Source: CAD feature listing. Evaluate the final solid. Frame: model axes, mm. A direction names the side the tool comes from. Round coordinates to 2 decimals unless told otherwise and drop trailing zeros. Loops run counter-clockwise (first coordinate to the right, second up) from the corner with the lowest first, then second, coordinate; pieces in that order, holes last.
(1) Section A-A, the plane y = 5. Return the cut outline in (x, z).
(2) First-contact query: pin 1 Ø6 at (x, z) = (18.5, 3) entering from +Y; pin 2 Ø4 at (x, y) = (53, 18) entering from +Z. Flat tips, straight axial feed; report the tip coordinate or a pass-through.
(3) Section C-C, the plane y = 36. Return the cut outline in (x, z), plus the area to 3 significant figures.
(4) Section B-B, the plane x = 54. Return the cut outline in (y, z).
(5) Material intervals for probe 1 along X at (y, z) = (50.25, 6); probe 2 along X at (y, z) = (19.5, 10.25); probe 3 along X at (y, z) = (51, 6), sorted ascending.
(6) Mould query, pull axis Z, two halves, no side actions, for faces 3 (the flat face through (33, 0, 6)), 4 (the flat face through (33, 22, 0)), 5 (the cylindrical face through (59.35, 49.88, 6.07)). Classes: pulls with the +Z half, pulls with the -Z half, needs draft (parallel to the pull), parting line crosses it, or undercut.
(7) Section D-D, the plane x = 34.5. Return the cut outline in (y, z), plus the area to 3 significant figures.
(8) Set-up query: faces 1 (the cylindrical face through (3.69, 49.88, 5)), 2 (the flat face through (33, 22, 12)). Return all of +Z, -Z, +X, -X, +Y, -Y with unobstructed straight access to the full face (end or side cutting, diameter ignored); none if empty.
```python
from build123d import *

# Parameters (mm, degrees)
SKETCH_1_W             = 66
SKETCH_1_H             = 55
EXTRUDE_1_DEPTH        = 12
SKETCH_2_R             = 23
CUT_EXTRUDE_1_DEPTH    = 87.746757864
HOLE_WIZARD_M6_1_D     = 5
HOLE_WIZARD_M4_1_D     = 3.3
HOLE_WIZARD_M4_1_DEPTH = 10.1
HOLE_WIZARD_M4_1_TIP   = 0.991420021


with BuildPart() as part:
    # 草图1 → 凸台-拉伸1 (new body)
    with BuildSketch(Plane.XY):
        with Locations((33, 27.5)):
            Rectangle(SKETCH_1_W, SKETCH_1_H)
    extrude(amount=EXTRUDE_1_DEPTH)

    # 草图2 → 切除-拉伸1 (cut, through all)
    with BuildSketch(Plane.XY.offset(12)):
        with Locations((33, 55.1)):
            Circle(SKETCH_2_R)
    extrude(amount=-CUT_EXTRUDE_1_DEPTH, mode=Mode.SUBTRACT)

    # M6 螺纹孔1 (through all)
    with Locations(Plane.XY.offset(12)):
        with Locations((13, 18), (53, 18), (13, 5), (53, 5)):
            Hole(HOLE_WIZARD_M6_1_D / 2)

    # M4 螺纹孔1
    with Locations(Plane(origin=(0, 55, 0), x_dir=(-1, 0, 0), z_dir=(0, 1, 0))):
        with Locations((-5, 6), (-61, 6)):
            Hole(HOLE_WIZARD_M4_1_D / 2, depth=HOLE_WIZARD_M4_1_DEPTH)
            with Locations((0, 0, -(HOLE_WIZARD_M4_1_DEPTH + HOLE_WIZARD_M4_1_TIP / 2))):  # 118° drill point
                Cone(0, HOLE_WIZARD_M4_1_D / 2, HOLE_WIZARD_M4_1_TIP, mode=Mode.SUBTRACT)


solid = part.part
```
Output values:
1. outline: (0, 0) - (10.5, 0) - (10.5, 12) - (0, 12) - close; (15.5, 0) - (50.5, 0) - (50.5, 12) - (15.5, 12) - close; (55.5, 0) - (66, 0) - (66, 12) - (55.5, 12) - close
2. pin 1: stops at y = 40.18
2. pin 2: passes through
3. outline: (0, 0) - (20.19, 0) - (20.19, 12) - (0, 12) - close; (45.81, 0) - (66, 0) - (66, 12) - (45.81, 12) - close
3. area: 484 mm2
4. outline: (0, 0) - (2.71, 0) - (2.71, 12) - (0, 12) - close; (7.29, 0) - (15.71, 0) - (15.71, 12) - (7.29, 12) - close; (20.29, 0) - (45.72, 0) - (45.72, 12) - (20.29, 12) - close
5. probe 1: x = 0 to 3.35, 6.65 to 10.52, 55.48 to 59.35, 62.65 to 66
5. probe 2: x = 0 to 11, 15 to 51, 55 to 66
5. probe 3: x = 0 to 3.35, 6.65 to 10.37, 55.63 to 59.35, 62.65 to 66
6. face 3: needs draft
6. face 4: pulls with the -Z half
6. face 5: undercut
7. outline: (0, 0) - (32.15, 0) - (32.15, 12) - (0, 12) - close
7. area: 386 mm2
8. face 1: +Y
8. face 2: +Z, +X, -X, +Y, -Y
